Source: three-view drawing plus pictorial views. Frame: mm from the lowest corner of the part. Coordinates: 2 decimals unless noted, no trailing zeros. Write each loop counter-clockwise with the first axis right and the second up, starting at its lowest first coordinate (ties: lowest second). Pieces come first, ordered by that corner, then holes. Notation, with made-up numbers: (47, 56) - (54, 56) arc R13 ccw to (54, 69) - close; hole circle Ø4 at (5, -15.75). An arc over 180 degrees is marked (long way). One line per item, written item: value.
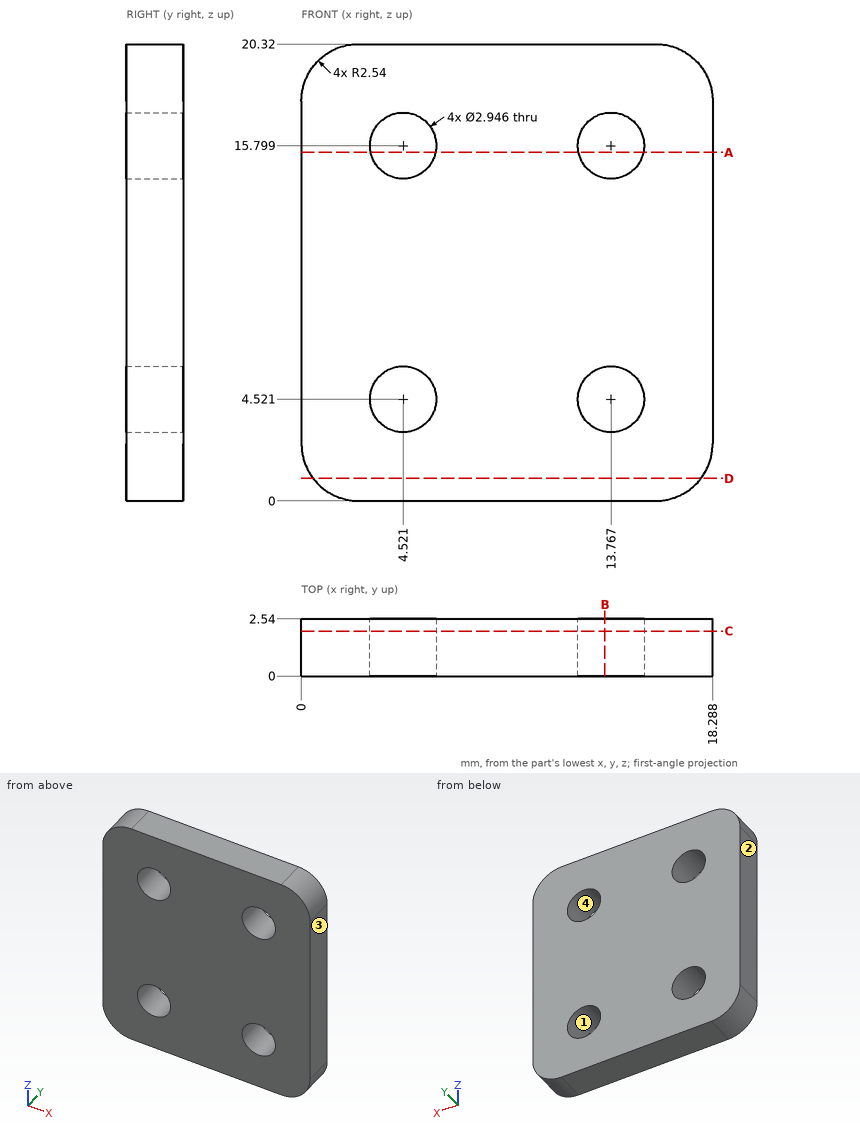
1) Section query B-B on x = 13.5. Output: boundary loops of the cut face in (y, z), then the cut area to 3 significant figures.
Values found:
outline: (0, 0) - (2.54, 0) - (2.54, 3.07) - (0, 3.07) - close; (0, 5.97) - (2.54, 5.97) - (2.54, 14.35) - (0, 14.35) - close; (0, 17.25) - (2.54, 17.25) - (2.54, 20.32) - (0, 20.32) - close
area: 36.9 mm2
2) Section query A-A on z = 15.5. Output: boundary loops of the cut face in (x, y) (1 decimal), then the cut area to 3 significant figures.
Values found:
outline: (0, 0) - (3.1, 0) - (3.1, 2.5) - (0, 2.5) - close; (6, 0) - (12.3, 0) - (12.3, 2.5) - (6, 2.5) - close; (15.2, 0) - (18.3, 0) - (18.3, 2.5) - (15.2, 2.5) - close
area: 31.8 mm2
3) Material intervals for line 1 (X direction, y = 0.3, z = 4) (1 decimal); line 2 (Z direction, x = 5.75, y = 1.85) (1 decimal); line 3 (Z direction, x = 4.25, y = 1.15), sorted ascending.
Values found:
line 1: 0 to 3.1, 5.9 to 12.4, 15.1 to 18.3
line 2: 0 to 3.7, 5.3 to 15, 16.6 to 20.3
line 3: 0 to 3.07, 5.97 to 14.35, 17.25 to 20.32
4) Contact query for a flat-ended pin moving along its axis: P1, Ø1.8, axis at x = 4.52, z = 4.52, coming from the +Y side. Output: stop coordinate, or through.
Values found:
P1: through
5) Section query C-C on y = 2. Output: boundary loops of the cut face in (x, z) (1 decimal).
Values found:
outline: (0, 2.5) arc R2.5 ccw to (2.5, 0) - (15.7, 0) arc R2.5 ccw to (18.3, 2.5) - (18.3, 17.8) arc R2.5 ccw to (15.7, 20.3) - (2.5, 20.3) arc R2.5 ccw to (0, 17.8) - close; hole circle Ø2.9 at (4.5, 4.5); hole circle Ø2.9 at (4.5, 15.8); hole circle Ø2.9 at (13.8, 4.5); hole circle Ø2.9 at (13.8, 15.8)
6) Draft query along X for the marked faces 1, 2, 3 and 4. Return one class per face: released by +X, released by -X, zero draft, split by the parting line, or undercut.
Values found:
face 1: undercut
face 2: released by -X
face 3: released by +X
face 4: undercut
7) Section query D-D on z = 1. Output: boundary loops of the cut face in (x, y), then the cut area to 3 significant figures.
Values found:
outline: (0.52, 0) - (17.77, 0) - (17.77, 2.54) - (0.52, 2.54) - close
area: 43.8 mm2
